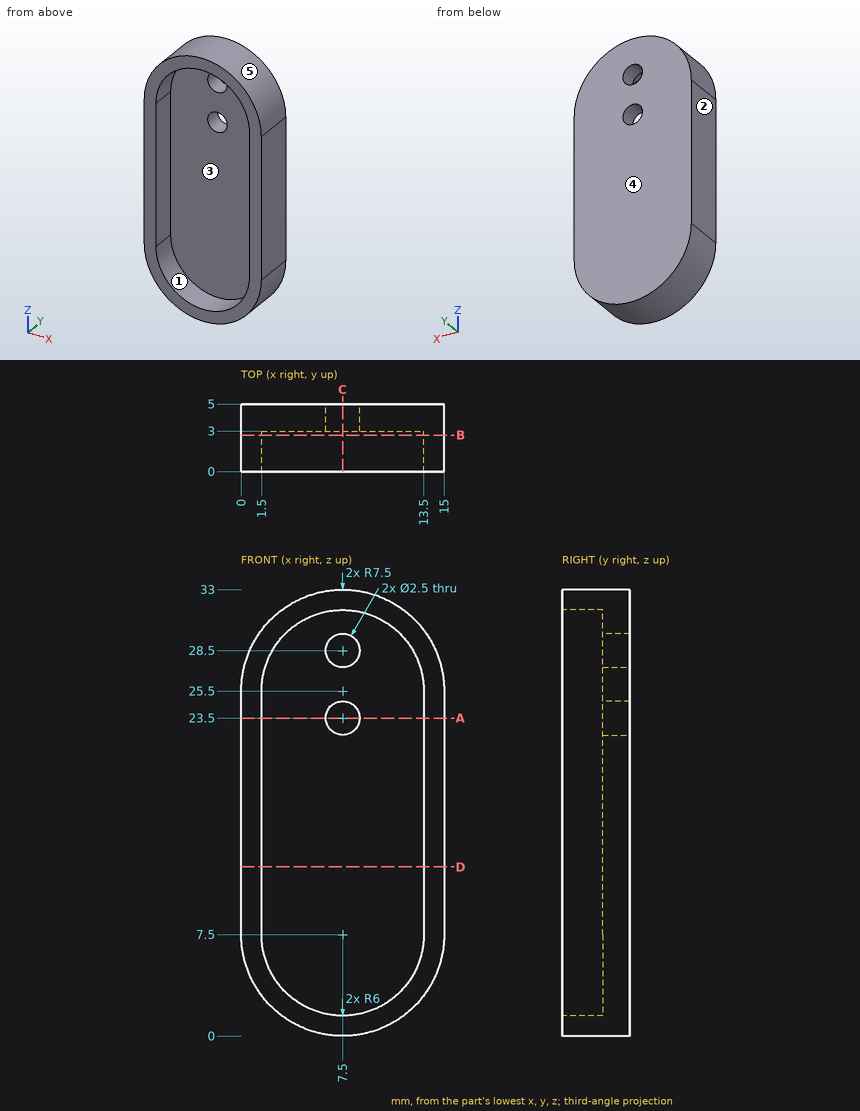
Geometry: see drawing. Coordinates: mm, zero at the bounding-box minimum. A direction names the side the tool comes from. Give positions to 0.01 mm unless a question says otherwise; leave off trailing zeros. Loops run counter-clockwise (first coordinate to the right, second up) from the corner with the lowest first, then second, coordinate; pieces in that order, holes last. Notation, with made-up numbers: (18, -12) -> (49, -12) arc R28 cw to (49, 7) -> close; hole circle Ø7 at (72.5, 56). An arc over 180 degrees is marked (long way). Put each result on its own line as item: value.
1. Cut plane D-D (z = 12.5). Return the cut outline in (x, y).
Taken from the geometry:
outline: (0, 0) -> (1.5, 0) -> (1.5, 3) -> (13.5, 3) -> (13.5, 0) -> (15, 0) -> (15, 5) -> (0, 5) -> close
2. Pin query (flat end, axial travel): P1, Ø6, axis at x = 5, z = 15.5, coming from the -Y side. Return the tip coordinate at first contact, or that it passes through.
Taken from the geometry:
P1: stops at y = 3
3. Pull-direction query (Z, two-part tool) for the marked faces 3, 4 and 5; classes: released by +Z, released by -Z, zero draft, split by the parting line, or undercut.
Taken from the geometry:
face 3: undercut
face 4: zero draft
face 5: released by +Z
4. Cut plane A-A (z = 23.5). Return the cut outline in (x, y).
Taken from the geometry:
outline: (0, 0) -> (1.5, 0) -> (1.5, 3) -> (6.25, 3) -> (6.25, 5) -> (0, 5) -> close; (8.75, 3) -> (13.5, 3) -> (13.5, 0) -> (15, 0) -> (15, 5) -> (8.75, 5) -> close
5. Cut plane C-C (x = 7.5). Return the cut outline in (y, z).
Taken from the geometry:
outline: (0, 0) -> (5, 0) -> (5, 22.25) -> (3, 22.25) -> (3, 1.5) -> (0, 1.5) -> close; (0, 31.5) -> (3, 31.5) -> (3, 29.75) -> (5, 29.75) -> (5, 33) -> (0, 33) -> close; (3, 24.75) -> (5, 24.75) -> (5, 27.25) -> (3, 27.25) -> close
6. Ray query, line 1 along X through (y, z) = (4.6, 23.5); line 2 along X through (y, z) = (1.85, 18); line 3 along Y through (x, z) = (4.5, 21). Return the intervals inside material, ascending. Write a range as [from, to].
Taken from the geometry:
line 1: x = [0, 6.25], [8.75, 15]
line 2: x = [0, 1.5], [13.5, 15]
line 3: y = [3, 5]
7. Cut plane B-B (y = 2.7). Return the cut outline in (x, z).
Taken from the geometry:
outline: (0, 7.5) arc R7.5 ccw to (15, 7.5) -> (15, 25.5) arc R7.5 ccw to (0, 25.5) -> close; hole (1.5, 7.5) arc R6 ccw to (13.5, 7.5) -> (13.5, 25.5) arc R6 ccw to (1.5, 25.5) -> close
8. Set-up query: the marked faces 1 and 2. Return all of +Z, -Z, +X, -X, +Y, -Y with unobstructed straight access to the full face (end or side cutting, diameter ignored); none if empty.
Taken from the geometry:
face 1: -Y
face 2: +Z, -Z, -X, +Y, -Y
